Source: three-view drawing plus pictorial views. Frame: mm from the lowest corner of the part. A direction names the side the tool comes from. Give positions to 0.01 mm unless a question says otherwise; leave off trailing zeros. Loops run counter-clockwise (first coordinate to the right, second up) from the corner with the lowest first, then second, coordinate; pieces in that order, holes last. Notation, with made-up numbers: (81.5, 52) - (118.5, 52) arc R20 cw to (118.5, 59) - close; hole circle Ø4 at (-5.75, 16). An arc over 180 degrees is marked (long way). Put each result on its own line as item: value.
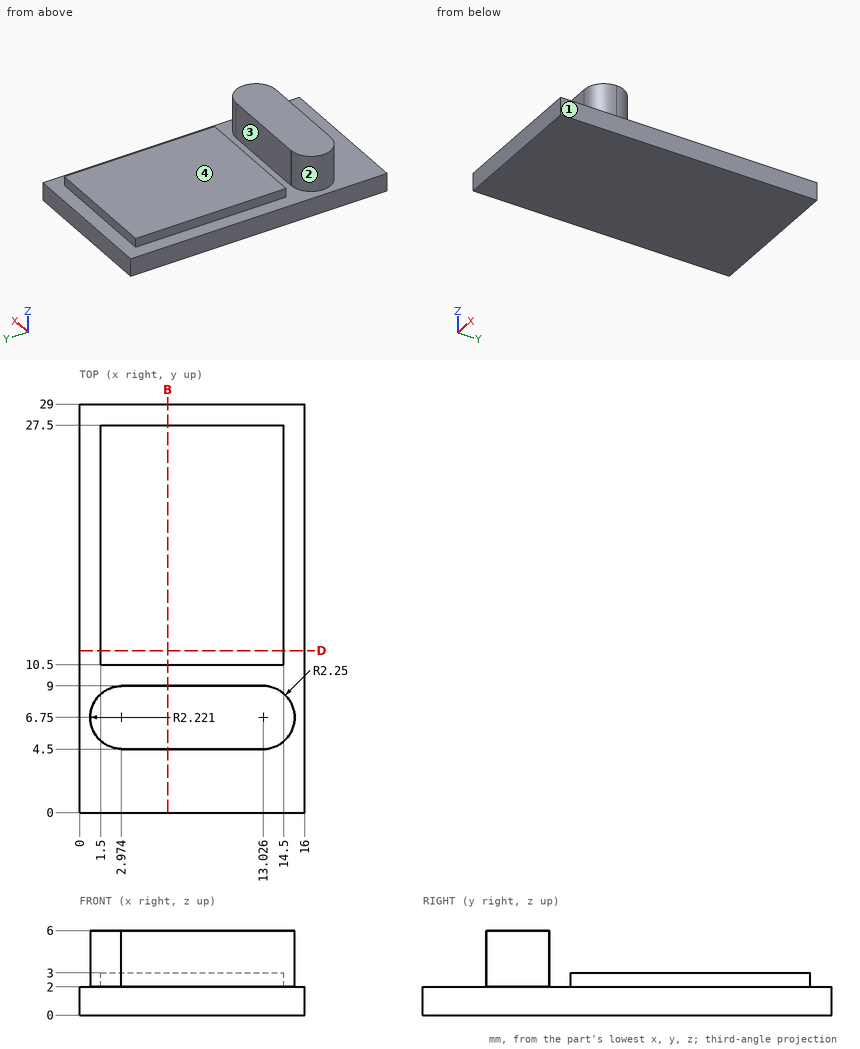
1) Pin query (flat end, axial travel): P1, Ø5, axis at x = 10, y = 17.5, coming from the +Z side; P2, Ø2, axis at x = 8.5, z = 3.5, coming from the +Y side. Return the tip coordinate at first contact, or that it passes through.
Check result:
P1: z = 3
P2: y = 27.5
2) Access query for the marked faces 1 and 2. Directions: +Z, -Z, +X, -X, +Y, -Y. A direction counts if a zero-diameter tool reaches every point of the face in a straight line with its end or side. Return the directions, or none.
Check result:
face 1: +Z, -Z, +X, +Y, -Y
face 2: +Z, -X
3) Mould query, pull axis Y, two halves, no side actions, for the marked faces 3 and 4. Classes: pulls with the +Y half, pulls with the -Y half, needs draft (parallel to the pull), parting line crosses it, or undercut.
Check result:
face 3: undercut
face 4: needs draft
4) Section query B-B, the plane x = 6.25. Output: boundary loops of the cut face in (y, z).
Check result:
outline: (0, 0) - (29, 0) - (29, 2) - (27.5, 2) - (27.5, 3) - (10.5, 3) - (10.5, 2) - (9, 2) - (9, 6) - (4.5, 6) - (4.5, 2) - (0, 2) - close
5) Material intervals for line 1 along Y through (x, z) = (6.5, 4.4); line 2 along Z through (x, y) = (10.75, 17.75); line 3 along Z through (x, y) = (1, 3.75), sorted ascending. Write a range as [from, to].
Check result:
line 1: [4.5, 9]
line 2: [0, 3]
line 3: [0, 2]
6) Section query D-D, the plane y = 11.5. Output: boundary loops of the cut face in (x, z).
Check result:
outline: (0, 0) - (16, 0) - (16, 2) - (14.5, 2) - (14.5, 3) - (1.5, 3) - (1.5, 2) - (0, 2) - close
